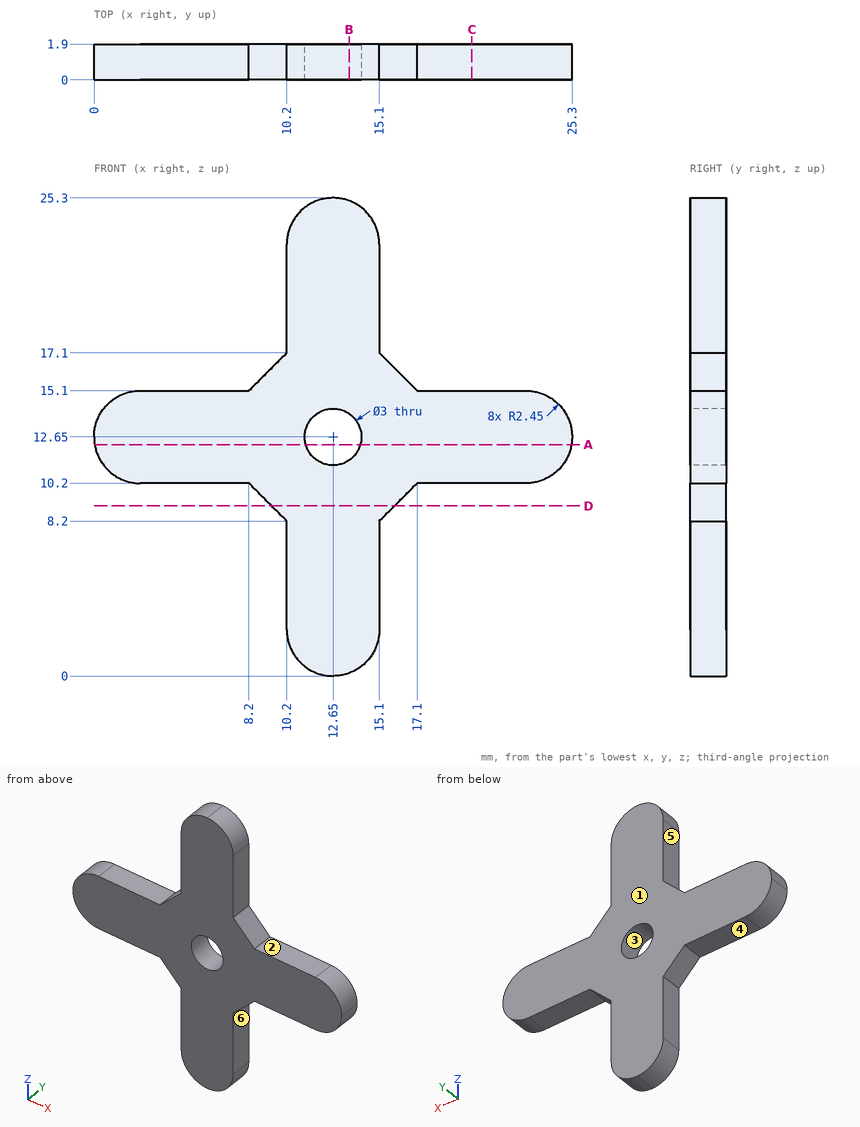
Geometry: see drawing. Coordinates: mm, zero at the bounding-box minimum. A direction names the side the tool comes from. Round coordinates to 2 decimals unless told otherwise and drop trailing zeros. Order: outer loops, then holes, each group sorted by start corner. A loop starts at its lowest first (then second) coordinate and runs counter-clockwise, first axis right, second up. Notation, with made-up numbers: (63, -6.75) -> (115, -6.75) arc R36 ccw to (115, 30.25) -> close; hole circle Ø10 at (63, 59). An arc over 180 degrees is marked (long way). Write each question's results on one line, items separated by ' | '.
Q1. Section query B-B (x = 13.5). Output: boundary loops of the cut face in (y, z) (1 decimal).
Response values:
outline: (0, 0.2) -> (1.9, 0.2) -> (1.9, 11.4) -> (0, 11.4) -> close; (0, 13.9) -> (1.9, 13.9) -> (1.9, 25.1) -> (0, 25.1) -> close
Q2. Pull-direction query (Z, two-part tool) for the marked faces 1, 2 and 3; classes: released by +Z, released by -Z, zero draft, split by the parting line, or undercut.
Response values:
face 1: zero draft | face 2: released by +Z | face 3: undercut
Q3. Section query C-C (x = 20). Output: boundary loops of the cut face in (y, z).
Response values:
outline: (0, 10.2) -> (1.9, 10.2) -> (1.9, 15.1) -> (0, 15.1) -> close
Q4. Section query D-D (z = 9). Output: boundary loops of the cut face in (x, y).
Response values:
outline: (9.4, 0) -> (15.9, 0) -> (15.9, 1.9) -> (9.4, 1.9) -> close
Q5. Section query A-A (z = 12.25). Output: boundary loops of the cut face in (x, y) (1 decimal).
Response values:
outline: (0, 0) -> (11.2, 0) -> (11.2, 1.9) -> (0, 1.9) -> close; (14.1, 0) -> (25.3, 0) -> (25.3, 1.9) -> (14.1, 1.9) -> close
Q6. Access query for the marked faces 4, 5 and 6. Directions: +Z, -Z, +X, -X, +Y, -Y. A direction counts if a zero-diameter tool reaches every point of the face in a straight line with its end or side. Return the directions, or none.
Response values:
face 4: -Z, -X, +Y, -Y | face 5: +Z, -X, +Y, -Y | face 6: -Z, +X, +Y, -Y
Q7. Ray query, line 1 along Z through (x, y) = (12.65, 1.2); line 2 along X through (y, z) = (1.25, 6). Return the intervals inside material, ascending.
Response values:
line 1: 0 to 11.15, 14.15 to 25.3 | line 2: 10.2 to 15.1
Q8. Pin query (flat end, axial travel): pin 1 Ø0.6 at (y, z) = (1, 5) entering from -X; pin 2 Ø2.5 at (x, z) = (12.65, 12.65) entering from -Y; pin 3 Ø0.6 at (x, y) = (6.5, 0.5) entering from -Z. Return the tip coordinate at first contact, or that it passes through.
Response values:
pin 1: x = 10.2 | pin 2: through | pin 3: z = 10.2
